Autodesk Inventor part; units mm, degrees
ref_plane "YZ Plane" through (0, 0, 0) normal (1, 0, 0) x (0, 1, 0)
ref_plane "XZ Plane" through (0, 0, 0) normal (0, 1, 0) x (-1, 0, 0)
ref_plane "XY Plane" through (0, 0, 0) normal (0, 0, 1) x (1, 0, 0)
sketch "Sketch1" plane through (0, 0, 0) normal (0, 0, 1) x (1, 0, 0)
  line L0 (0, 0) -> (20, 0)
  line L1 (20, 0) -> (20, 10)
  line L2 (20, 10) -> (0, 10)
  line L3 (0, 10) -> (0, 0)
  dimension "d0" = 20
  dimension "d1" = 10
sketch "Sketch1 outline for Extrusion1" plane through (0, 0, 0) normal (0, 0, 1) x (1, 0, 0)
  line L0 (0, 0) -> (20, 0)
  line L1 (0, 10) -> (0, 0)
  line L2 (20, 10) -> (0, 10)
  line L3 (20, 0) -> (20, 10)
extrude "Extrusion1" add sketch "Sketch1 outline for Extrusion1" along normal blind 4
sketch "Sketch2" plane through (0, 0, 4) normal (0, 0, 1) x (1, 0, 0)
  line L0 (0, 10) -> (0, 0)
  line L1 (0, 5) -> (7.071, 5)
  line L2 (7.071, 5) -> (14.142, 5)
  circle A0 centre (7.071, 5) radius 1.6
  circle A1 centre (14.142, 5) radius 2.95
  dimension "d4" = 7.071
  dimension "d5" = 7.071
  dimension "d6" = 3.2
  dimension "d7" = 5.9
sketch "Sketch2 outline for Extrusion2" plane through (0, 0, 4) normal (0, 0, 1) x (1, 0, 0)
  circle A0 centre (7.071, 5) radius 1.6
extrude "Extrusion2" cut sketch "Sketch2 outline for Extrusion2" against normal blind 4
sketch "Sketch3" plane through (0, 0, 4) normal (0, 0, 1) x (1, 0, 0)
  circle A0 centre (7.071, 5) radius 1.6
  line L0 (7.071, 5) -> (14.142, 5)
  circle A1 centre (14.142, 5) radius 1.6
  point P0 (0, 0)
  dimension "d10" = 7.071
  dimension "d11" = 3.2
sketch "Sketch3 outline for Extrusion3" plane through (0, 0, 4) normal (0, 0, 1) x (1, 0, 0)
  circle A0 centre (14.142, 5) radius 1.6
extrude "Extrusion3" cut sketch "Sketch3 outline for Extrusion3" against normal blind 3
sketch "Sketch5" plane through (0, 0, 4) normal (0, 0, 1) x (1, 0, 0)
  line L0 (0, 0) -> (20, 0)
  line L1 (0, 10) -> (4, 10)
  line L2 (4, 10) -> (4, 0)
  line L3 (4, 0) -> (0, 0)
  line L4 (0, 0) -> (0, 10)
  dimension "d17" = 4
sketch "Sketch5 outline for Extrusion5" plane through (0, 0, 4) normal (0, 0, 1) x (1, 0, 0)
  line L0 (4, 10) -> (0, 10)
  line L1 (4, 0) -> (4, 10)
  line L2 (0, 0) -> (4, 0)
  line L3 (0, 10) -> (0, 0)
extrude "Extrusion5" cut sketch "Sketch5 outline for Extrusion5" against normal blind 4
sketch "Sketch6" plane through (0, 0, 4) normal (0, 0, 1) x (1, 0, 0)
  circle A0 centre (7.071, 5) radius 1.6
  line L0 (7.071, 5) -> (9.899427, 7.828427)
  line L1 (7.071, 5) -> (11.071, 5) construction
  line L2 (20, 10) -> (4, 10)
  line L3 (4, 0) -> (20, 0)
  line L4 (7.071, 5) -> (5.414, 5)
  line L5 (5.414, 5) -> (8.242427, 7.828427)
  line L6 (5.414, 5) -> (9.414, 5) construction
  line L7 (5.414, 5) -> (10.414, 0)
  line L8 (5.414, 5) -> (12.485068, 5) construction
  arc A1 (8.242427, 7.828427) -> (8.242427, 2.171573) centre (11.070854, 5) ccw
  circle A2 centre (7.071, 5) radius 1.6
  line L9 (20, 10) -> (4, 10)
  arc A3 (8.914, 10) -> (10.414, 0) centre (9.664, 5) ccw
  line L10 (8.914, 10) -> (4, 10)
  line L11 (4, 10) -> (4, 0)
  line L12 (4, 0) -> (8.914, 0)
  line L13 (8.914, 0) -> (8.914, 10)
  line L14 (7.071, 5) -> (12.071, 0)
  line L15 (4, 0) -> (20, 0)
  line L16 (7.071, 5) -> (14.142068, 5) construction
  line L17 (9.899427, 7.828427) -> (12.071, 10)
  arc A4 (9.899427, 7.828427) -> (9.899427, 2.171573) centre (12.727854, 5) ccw
  line L18 (8.242427, 7.828427) -> (10.414, 10)
  point P0 (0, 0)
  point P1 (13.001674, 10)
  point P2 (10.571, 0)
  point P3 (9.364849, 1.723072)
  point P4 (8.914, 10)
  point P5 (8.914, 0)
  point P6 (7.390866, 3.432299)
  point P7 (5.472054, 4.941946)
  point P8 (5.472054, 5.058054)
  point P9 (7.390866, 6.567701)
  point P10 (7.012946, 3.401054)
  point P11 (8.914, 1.5)
  point P12 (8.914, 0)
  point P13 (8.914, 10)
  point P14 (8.914, 8.5)
  dimension "d21" = 4
  dimension "d22" = 45
  dimension "d24" = 1.657
  dimension "d25" = 45
  dimension "d26" = 45
  dimension "d27" = 4
  dimension "d35" = 45
  dimension "d36" = 4
sketch "Sketch6 outline for Extrusion6" plane through (0, 0, 4) normal (0, 0, 1) x (1, 0, 0)
  line L0 (5.472054, 4.941946) -> (5.414, 5)
  line L1 (5.414, 5) -> (5.472054, 5.058054)
  arc A0 (5.472054, 5.058054) -> (5.472054, 4.941946) centre (7.071, 5) cw
  line L2 (12.071, 10) -> (4, 10)
  line L3 (4, 10) -> (4, 0)
  line L4 (4, 0) -> (12.071, 0)
  line L5 (12.071, 0) -> (9.899427, 2.171573)
  arc A1 (9.899427, 2.171573) -> (9.899427, 7.828427) centre (12.727854, 5) cw
  line L6 (9.899427, 7.828427) -> (12.071, 10)
extrude "Extrusion6" add sketch "Sketch6 outline for Extrusion6" along normal blind 5
sketch "Sketch8" plane through (0, 0, 0) normal (0, 0, -1) x (-1, 0, 0)
  circle A0 centre (-14.142, 5) radius 1.6
  circle A1 centre (-14.142, 5) radius 2.95
  point P0 (0, 0)
  dimension "d37" = 5.9
sketch "Sketch8 outline for Extrusion8" plane through (0, 0, 0) normal (0, 0, -1) x (-1, 0, 0)
  circle A0 centre (-14.142, 5) radius 2.95
extrude "Extrusion8" cut sketch "Sketch8 outline for Extrusion8" against normal blind 3
sketch "Sketch9" plane through (0, 0, 0) normal (0, 0, -1) x (-1, 0, 0)
  arc A0 (-5.472054, 5.058054) -> (-5.472054, 4.941946) centre (-7.071, 5) ccw
  circle A1 centre (-7.071, 5) radius 2.95
  point P0 (0, 0)
  dimension "d40" = 5.9
sketch "Sketch9 outline for Extrusion9" plane through (0, 0, 0) normal (0, 0, -1) x (-1, 0, 0)
  circle A0 centre (-7.071, 5) radius 2.95
extrude "Extrusion9" cut sketch "Sketch9 outline for Extrusion9" against normal blind 3.9
sketch "Sketch10" plane through (0, 0, 9) normal (0, 0, 1) x (1, 0, 0)
  arc A0 (5.472054, 4.941946) -> (5.472054, 5.058054) centre (7.071, 5) ccw
  circle A1 centre (7.071, 5) radius 1.6
  point P0 (0, 0)
  point P1 (5.472054, 5.058054)
sketch "Sketch10 outline for Extrusion10" plane through (0, 0, 9) normal (0, 0, 1) x (1, 0, 0)
  arc A0 (5.472054, 5.058054) -> (5.472054, 4.941946) centre (7.071, 5) ccw
  arc A1 (5.472054, 4.941946) -> (5.472054, 5.058054) centre (7.071, 5) ccw
extrude "Extrusion10" add sketch "Sketch10 outline for Extrusion10" against normal blind 5.1
sketch "Sketch11" plane through (12.071, 10, 9) normal (0, 1, 0) x (1, 0, 0)
  line L0 (-8.071, 0) -> (-8.071, 9)
  line L1 (7.929, 9) -> (7.929, 5)
  line L2 (-8.071, 9) -> (7.929, 9)
  line L3 (7.929, 9) -> (7.929, 5)
  line L4 (7.929, 5) -> (-8.071, 5)
  line L5 (-8.071, 5) -> (-8.071, 9)
  point P0 (-12.071, 9)
sketch "Sketch11 outline for Extrusion11" plane through (12.071, 10, 9) normal (0, 1, 0) x (1, 0, 0)
  line L0 (7.929, 9) -> (-8.071, 9)
  line L1 (7.929, 5) -> (7.929, 9)
  line L2 (-8.071, 5) -> (7.929, 5)
  line L3 (-8.071, 9) -> (-8.071, 5)
extrude "Extrusion11" add sketch "Sketch11 outline for Extrusion11" along normal blind 5
sketch "Sketch12" plane through (20, 0, 0) normal (0, -1, 0) x (1, 0, 0)
  line L0 (0, 4) -> (0, 0)
  line L1 (-7.929, 4) -> (-16, 4)
  line L2 (0, 0) -> (-16, 0)
  line L3 (-16, 0) -> (-16, 4)
  line L4 (-16, 4) -> (0, 4)
  line L5 (0, 4) -> (0, 0)
  point P0 (-20, 0)
sketch "Sketch12 outline for Extrusion12" plane through (20, 0, 0) normal (0, -1, 0) x (1, 0, 0)
  line L0 (-16, 4) -> (-16, 0)
  line L1 (-7.929, 4) -> (-16, 4)
  line L2 (0, 4) -> (-7.929, 4)
  line L3 (0, 0) -> (0, 4)
  line L4 (-16, 0) -> (0, 0)
extrude "Extrusion12" add sketch "Sketch12 outline for Extrusion12" along normal blind 5
sketch "Sketch13" plane through (0, 0, 4) normal (0, 0, 1) x (1, 0, 0)
  line L0 (9.899427, 2.171573) -> (12.071, 0)
  line L1 (12.071, 10) -> (9.899427, 7.828427)
  line L2 (12.071, 10) -> (17.071, 15)
  line L3 (20, 15) -> (4, 15)
  line L4 (12.071, 10) -> (19.142068, 10) construction
  line L5 (20, 15) -> (20, -5)
  line L6 (12.071, 10) -> (4, 10)
  line L7 (4, 10) -> (17.071, 10)
  line L8 (17.071, 10) -> (17.071, 15)
  line L9 (17.071, 15) -> (4, 15)
  line L10 (4, 15) -> (4, 10)
  line L11 (12.071, 0) -> (17.071, -5)
  line L12 (12.071, 0) -> (19.142068, 0) construction
  line L13 (4, 0) -> (12.071, 0)
  line L14 (4, 0) -> (20, 0)
  line L15 (20, 0) -> (20, -5)
  line L16 (20, -5) -> (4, -5)
  line L17 (4, -5) -> (4, 0)
  dimension "d50" = 45
  dimension "d51" = 45
sketch "Sketch13 outline for Extrusion13" plane through (0, 0, 4) normal (0, 0, 1) x (1, 0, 0)
  line L0 (4, 15) -> (4, 10)
  line L1 (17.071, 15) -> (4, 15)
  line L2 (12.071, 10) -> (17.071, 15)
  line L3 (4, 10) -> (12.071, 10)
  line L4 (4, 0) -> (4, -5)
  line L5 (12.071, 0) -> (4, 0)
  line L6 (17.071, -5) -> (12.071, 0)
  line L7 (4, -5) -> (17.071, -5)
extrude "Extrusion13" add sketch "Sketch13 outline for Extrusion13" along normal blind 5
fillet "Fillet2" radius 4 4 edges at (20, 15, 2) (4, 15, 4.5) (20, -5, 2) (4, -5, 4.5)
fillet "Fillet3" radius 1 2 edges at (16.9553, 14.8843, 6.5) (16.9553, -4.8843, 6.5)
properties part number "corner fitter"
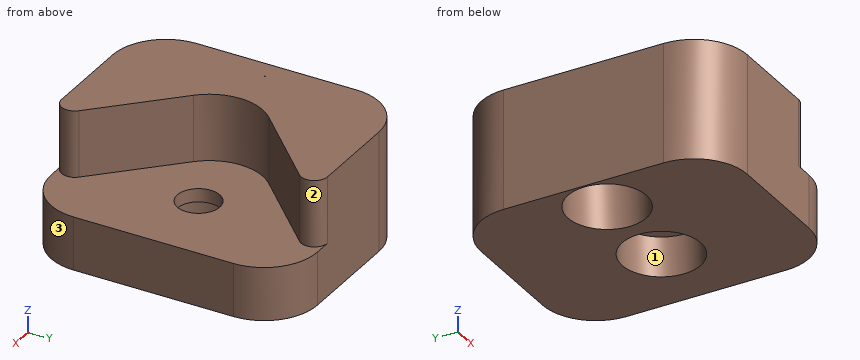
Model file for the job. Use its own axes, mm. Face numbers are marked on the shaded views. A direction names the side the tool comes from. Give positions to 0.01 mm unless a question says otherwise; leave off trailing zeros. Loops run counter-clockwise (first coordinate to the right, second up) from the corner with the lowest first, then second, coordinate; pieces in that order, holes last. Notation, with made-up numbers: (47.25, 11) -> (60.25, 11) arc R29 ccw to (60.25, 38) -> close; hole circle Ø1 at (63.25, 79.5). An arc over 180 degrees is marked (long way). Use a Markdown table: item, result. Add a question column.
(1) Slice it at A-A on z = 4.25. List the corners of the cut face in (x, y).
(2) Slice it at C-C on z = 2.75. List the corners of the cut face in (x, y).
(3) Slice it at D-D on y = 4. List the corners of the cut face in (x, z), and give its area (3 significant figures).
(4) Tool access for the marked faces 1, 2 and 3: list every direction of +Z, -Z, +X, -X, +Y, -Y with a clear straight run to the whole face (end or side of a thin tool).
(5) Slice it at B-B on x = 13.25. List the corners of the cut face in (y, z), and give its area (3 significant figures).
(6) Wall check: line 1 along Y through (x, z) = (15, 1.25); line 2 along X through (y, z) = (3.25, 1.75); line 3 along Y through (x, z) = (10.25, 6.5). Give the ranges that are in metal, low to high.
(7) Drop flat-ended pins along their axis: pin 1 Ø3 at (x, y) = (7, 4.5) entering from -Z; pin 2 Ø3 at (x, y) = (14.142, 5) entering from -Z; pin 3 Ø5.5 at (x, y) = (14.142, 5) entering from -Z. Give the stop position or say it passes through.
Filled sheet:
| question | item | result |
|---|---|---|
| 1 | outline | (4, -1) arc R4 ccw to (8, -5) -> (14.66, -5) arc R1 ccw to (15.36, -3.29) -> (9.9, 2.17) arc R4 cw to (9.9, 7.83) -> (15.36, 13.29) arc R1 ccw to (14.66, 15) -> (8, 15) arc R4 ccw to (4, 11) -> close; hole (5.41, 5) -> (5.47, 4.94) arc R1.6 cw to (5.47, 5.06) -> close |
| 2 | outline | (4, -1) arc R4 ccw to (8, -5) -> (16, -5) arc R4 ccw to (20, -1) -> (20, 11) arc R4 ccw to (16, 15) -> (8, 15) arc R4 ccw to (4, 11) -> close; hole circle Ø5.9 at (7.07, 5); hole circle Ø5.9 at (14.14, 5) |
| 3 | outline | (4, 0) -> (4.3, 0) -> (4.3, 3.9) -> (9.85, 3.9) -> (9.85, 0) -> (11.37, 0) -> (11.37, 3) -> (12.89, 3) -> (12.89, 4) -> (8.85, 4) -> (8.85, 9) -> (4, 9) -> close; (15.39, 3) -> (16.92, 3) -> (16.92, 0) -> (20, 0) -> (20, 4) -> (15.39, 4) -> close |
| 3 | area | 47.5 mm2 |
| 4 | face 1 | -Z |
| 4 | face 2 | +Z, +X |
| 4 | face 3 | +Z, -Z, +X, -Y |
| 5 | outline | (-5, 0) -> (2.19, 0) -> (2.19, 3) -> (3.67, 3) -> (3.67, 4) -> (-1.18, 4) -> (-1.18, 9) -> (-5, 9) -> close; (6.33, 3) -> (7.81, 3) -> (7.81, 0) -> (15, 0) -> (15, 9) -> (11.18, 9) -> (11.18, 4) -> (6.33, 4) -> close |
| 5 | area | 98.7 mm2 |
| 6 | line 1 | -5 to 2.18, 7.82 to 15 |
| 6 | line 2 | 4 to 4.7, 9.45 to 11.77, 16.52 to 20 |
| 6 | line 3 | -5 to 1.82, 8.18 to 15 |
| 7 | pin 1 | z = 3.9 |
| 7 | pin 2 | through |
| 7 | pin 3 | z = 3 |
